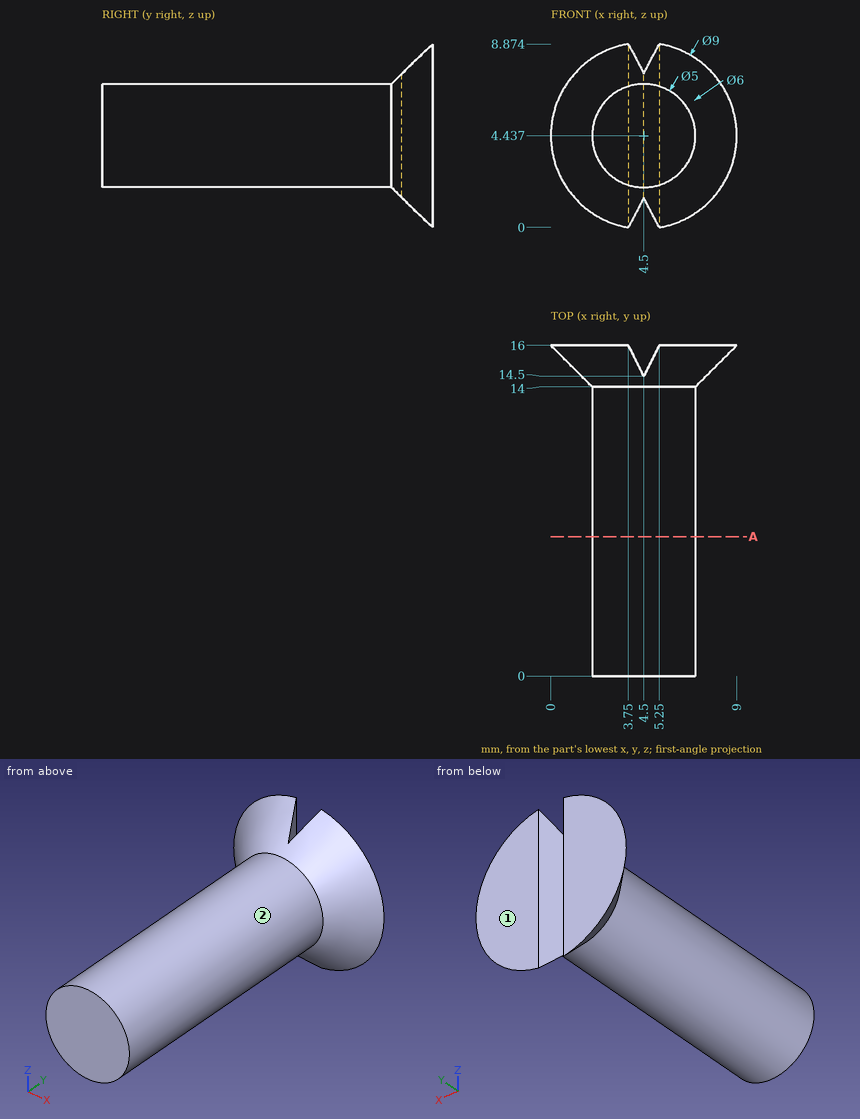
Geometry check sheet. Reference: drawing and pictorial views, mm from the part's lowest x, y, z. A direction names the side the tool comes from. Round coordinates to 2 decimals unless told otherwise and drop trailing zeros. Order: outer loops, then holes, each group sorted by start corner. A loop starts at its lowest first (then second) coordinate and runs counter-clockwise, first axis right, second up. Notation, with made-up numbers: M 70.5,-25 L 113.5,-25 A17 cw 113.5,-9 Z; hole C 60,56.25 d9. An arc over 180 degrees is marked long. Write item = value, one per line.
Q1. Scan lines: line 1 (Z direction, x = 4.25, y = 9.25); line 2 (Z direction, x = 2.5, y = 4); line 3 (Y direction, x = 1.5, z = 2.25). Record each from-to range of solid material in increasing order.
Answer block:
line_1 = 1.95 to 6.92
line_2 = 2.94 to 5.94
line_3 = 15.21 to 16
Q2. Depth check by flat-ended pin: pin 1 Ø4 at (x, y) = (7.5, 14) entering from +Z; pin 2 Ø4 at (x, y) = (1.5, 12) entering from -Z; pin 3 Ø3 at (y, z) = (11, 6.5) entering from +X. Enter the tip coordinate at first touch or a pass-through.
Answer block:
pin_1 = 8.17
pin_2 = 2.15
pin_3 = 6.94
Q3. Section check A-A (y = 6.75). Enter the section's corners in (x, z).
Answer block:
outline = C 4.5,4.44 d5
Q4. Set-up check for the marked faces 1 and 2: record each of +Z, -Z, +X, -X, +Y, -Y from which the full face is reachable in a straight line by a thin tool's end or side.
Answer block:
face_1 = +Z, -Z, +X, -X, +Y
face_2 = -Y
